For this review, take the finished solid that the model builds, in its own axes (mm). Give positions to 0.01 mm unless a question says otherwise; leave off trailing zeros. Loops run counter-clockwise (first coordinate to the right, second up) from the corner with the lowest first, then second, coordinate; pieces in that order, holes last. Notation, with made-up numbers: M 79,86 L 87,86 A26 ccw 87,103 Z; hole C 87,85 d9. An arc over 180 degrees is marked long. Use CSV: the item, a comma, the result in double quotes. Start each with the question number.
1. Insertion check: P1, Ø8, axis at x = 16.5, y = -30.5, coming from the -Z side; P2, Ø6, axis at x = 1.5, z = 7.5, coming from the -Y side; P3, Ø5, axis at y = 28.5, z = 10, coming from the -X side; P4, Ø8, axis at x = -27.5, y = -7.5, coming from the +Z side. Each pin has a flat end and moves straight along its axis. Give the tip position at first contact, or say it passes through.
2. Take a section at D-D, the plane y = -21. Write out the cut boundary in (x, z), and give its area (3 significant figures).
3. Take a section at A-A, the plane x = 0. Write out the cut boundary in (y, z) (3 decimals), and give its area (3 significant figures).
4. To check wall thickness, follow line 1 (Y direction, x = 0, z = 3.8) (3 decimals); line 2 (Z direction, x = 9.5, y = -13); line 3 (X direction, y = -36.5, z = 1.25). State the ranges of each line that lie inside material, in increasing order. Write a range as [from, to].
5. Take a section at C-C, the plane y = 2.5. Write out the cut boundary in (x, z).
from build123d import *

# Parameters (mm, degrees)
F1_DEPTH = 5.08
F2_R     = 3.6481835691
F3_DEPTH = 2.54
F4_R     = 1.6674700951
F5_DEPTH = 5.08
F6_R     = 8.255
F7_DEPTH = 25.4


with BuildPart() as f1:
    # F0 (on Top) → F1 (new body)
    with BuildSketch(Plane.XY):
        with BuildLine():
            ThreePointArc((37.7468732805, -5.1752833301), (38.0116158035, -2.5936584214), (38.1, 0))
            ThreePointArc((38.1, 0), (38.0577032994, 1.7947756344), (37.9309071088, 3.5855663298))
            Line((37.9309071088, 3.5855663298), (34.7138681986, 5.6416139149))
            Line((34.7138681986, 5.6416139149), (34.1414945044, -7.0454814325))
            Line((34.1414945044, -7.0454814325), (37.7468732805, -5.1752833301))
        make_face()
        with BuildLine():
            ThreePointArc((37.9309071088, 3.5855663298), (38.0577032994, 1.7947756344), (38.1, 0))
            ThreePointArc((38.1, 0), (38.0116158035, -2.5936584214), (37.7468732805, -5.1752833301))
            Line((37.7468732805, -5.1752833301), (45.4150282226, -1.1976239184))
            Line((45.4150282226, -1.1976239184), (37.9309071088, 3.5855663298))
        make_face()
        with BuildLine():
            Line((34.7138681986, 5.6416139149), (37.9309071088, 3.5855663298))
            ThreePointArc((37.9309071088, 3.5855663298), (36.4745263648, 11.0099467057), (33.5798171863, 18.0001632696))
            Line((33.5798171863, 18.0001632696), (31.7622793488, 14.3679527485))
            Line((31.7622793488, 14.3679527485), (24.7680518549, 24.9684613101))
            Line((24.7680518549, 24.9684613101), (28.5792054533, 25.1960118999))
            ThreePointArc((28.5792054533, 25.1960118999), (23.0370273887, 30.3464226737), (16.586412263, 34.3001593035))
            Line((16.586412263, 34.3001593035), (17.250953042, 30.2933173283))
            Line((17.250953042, 30.2933173283), (5.3616815377, 34.7582051315))
            Line((5.3616815377, 34.7582051315), (8.3112186861, 37.1824373052))
            ThreePointArc((8.3112186861, 37.1824373052), (0.8001669499, 38.0915966173), (-6.7424383934, 37.4986603029))
            Line((-6.7424383934, 37.4986603029), (-3.8496509884, 34.6476643207))
            Line((-3.8496509884, 34.6476643207), (-16.0926688901, 31.2714959807))
            Line((-16.0926688901, 31.2714959807), (-15.1313711312, 34.9664354444))
            ThreePointArc((-15.1313711312, 34.9664354444), (-21.7423300671, 31.2870753388), (-27.4959067505, 26.3739475992))
            Line((-27.4959067505, 26.3739475992), (-23.4798191861, 25.7677811734))
            Line((-23.4798191861, 25.7677811734), (-31.4001667715, 15.8401382443))
            Line((-31.4001667715, 15.8401382443), (-32.7942914728, 19.3944437094))
            ThreePointArc((-32.7942914728, 19.3944437094), (-35.9799959931, 12.5319546895), (-37.7468732805, 5.1752833301))
            Line((-37.7468732805, 5.1752833301), (-34.1414945044, 7.0454814325))
            Line((-34.1414945044, 7.0454814325), (-34.7138681986, -5.6416139149))
            Line((-34.7138681986, -5.6416139149), (-37.9309071088, -3.5855663298))
            ThreePointArc((-37.9309071088, -3.5855663298), (-36.4745263648, -11.0099467057), (-33.5798171863, -18.0001632696))
            Line((-33.5798171863, -18.0001632696), (-31.7622793488, -14.3679527485))
            Line((-31.7622793488, -14.3679527485), (-24.7680518549, -24.9684613101))
            Line((-24.7680518549, -24.9684613101), (-28.5792054533, -25.1960118999))
            ThreePointArc((-28.5792054533, -25.1960118999), (-23.0370273887, -30.3464226737), (-16.586412263, -34.3001593035))
            Line((-16.586412263, -34.3001593035), (-17.250953042, -30.2933173283))
            Line((-17.250953042, -30.2933173283), (-5.3616815377, -34.7582051315))
            Line((-5.3616815377, -34.7582051315), (-8.3112186861, -37.1824373052))
            ThreePointArc((-8.3112186861, -37.1824373052), (-0.8001669499, -38.0915966173), (6.7424383934, -37.4986603029))
            Line((6.7424383934, -37.4986603029), (3.8496509884, -34.6476643207))
            Line((3.8496509884, -34.6476643207), (16.0926688901, -31.2714959807))
            Line((16.0926688901, -31.2714959807), (15.1313711312, -34.9664354444))
            ThreePointArc((15.1313711312, -34.9664354444), (21.7423300671, -31.2870753388), (27.4959067505, -26.3739475992))
            Line((27.4959067505, -26.3739475992), (23.4798191861, -25.7677811734))
            Line((23.4798191861, -25.7677811734), (31.4001667715, -15.8401382443))
            Line((31.4001667715, -15.8401382443), (32.7942914728, -19.3944437094))
            ThreePointArc((32.7942914728, -19.3944437094), (35.9799959931, -12.5319546895), (37.7468732805, -5.1752833301))
            Line((37.7468732805, -5.1752833301), (34.1414945044, -7.0454814325))
            Line((34.1414945044, -7.0454814325), (34.7138681986, 5.6416139149))
        make_face()
        with BuildLine():
            Line((31.7622793488, 14.3679527485), (33.5798171863, 18.0001632696))
            ThreePointArc((33.5798171863, 18.0001632696), (31.2870753388, 21.7423300671), (28.5792054533, 25.1960118999))
            Line((28.5792054533, 25.1960118999), (24.7680518549, 24.9684613101))
            Line((24.7680518549, 24.9684613101), (31.7622793488, 14.3679527485))
        make_face()
        with BuildLine():
            ThreePointArc((28.5792054533, 25.1960118999), (31.2870753388, 21.7423300671), (33.5798171863, 18.0001632696))
            Line((33.5798171863, 18.0001632696), (37.4454753092, 25.7253857188))
            Line((37.4454753092, 25.7253857188), (28.5792054533, 25.1960118999))
        make_face()
        with BuildLine():
            Line((36.0375839551, -27.6631819246), (32.7942914728, -19.3944437094))
            ThreePointArc((32.7942914728, -19.3944437094), (30.3464226737, -23.0370273887), (27.4959067505, -26.3739475992))
            Line((27.4959067505, -26.3739475992), (36.0375839551, -27.6631819246))
        make_face()
        with BuildLine():
            ThreePointArc((27.4959067505, -26.3739475992), (30.3464226737, -23.0370273887), (32.7942914728, -19.3944437094))
            Line((32.7942914728, -19.3944437094), (31.4001667715, -15.8401382443))
            Line((31.4001667715, -15.8401382443), (23.4798191861, -25.7677811734))
            Line((23.4798191861, -25.7677811734), (27.4959067505, -26.3739475992))
        make_face()
        with BuildLine():
            Line((17.250953042, 30.2933173283), (16.586412263, 34.3001593035))
            ThreePointArc((16.586412263, 34.3001593035), (12.5319546895, 35.9799959931), (8.3112186861, 37.1824373052))
            Line((8.3112186861, 37.1824373052), (5.3616815377, 34.7582051315))
            Line((5.3616815377, 34.7582051315), (17.250953042, 30.2933173283))
        make_face()
        with BuildLine():
            ThreePointArc((8.3112186861, 37.1824373052), (12.5319546895, 35.9799959931), (16.586412263, 34.3001593035))
            Line((16.586412263, 34.3001593035), (15.1730235525, 42.8221723852))
            Line((15.1730235525, 42.8221723852), (8.3112186861, 37.1824373052))
        make_face()
        with BuildLine():
            Line((12.8950074891, -43.5623446725), (15.1313711312, -34.9664354444))
            ThreePointArc((15.1313711312, -34.9664354444), (11.0099467057, -36.4745263648), (6.7424383934, -37.4986603029))
            Line((6.7424383934, -37.4986603029), (12.8950074891, -43.5623446725))
        make_face()
        with BuildLine():
            ThreePointArc((6.7424383934, -37.4986603029), (11.0099467057, -36.4745263648), (15.1313711312, -34.9664354444))
            Line((15.1313711312, -34.9664354444), (16.0926688901, -31.2714959807))
            Line((16.0926688901, -31.2714959807), (3.8496509884, -34.6476643207))
            Line((3.8496509884, -34.6476643207), (6.7424383934, -37.4986603029))
        make_face()
        with BuildLine():
            Line((-3.8496509884, 34.6476643207), (-6.7424383934, 37.4986603029))
            ThreePointArc((-6.7424383934, 37.4986603029), (-11.0099467057, 36.4745263648), (-15.1313711312, 34.9664354444))
            Line((-15.1313711312, 34.9664354444), (-16.0926688901, 31.2714959807))
            Line((-16.0926688901, 31.2714959807), (-3.8496509884, 34.6476643207))
        make_face()
        with BuildLine():
            ThreePointArc((-15.1313711312, 34.9664354444), (-11.0099467057, 36.4745263648), (-6.7424383934, 37.4986603029))
            Line((-6.7424383934, 37.4986603029), (-12.8950074891, 43.5623446725))
            Line((-12.8950074891, 43.5623446725), (-15.1313711312, 34.9664354444))
        make_face()
        with BuildLine():
            Line((-15.1730235525, -42.8221723852), (-8.3112186861, -37.1824373052))
            ThreePointArc((-8.3112186861, -37.1824373052), (-12.5319546895, -35.9799959931), (-16.586412263, -34.3001593035))
            Line((-16.586412263, -34.3001593035), (-15.1730235525, -42.8221723852))
        make_face()
        with BuildLine():
            ThreePointArc((-16.586412263, -34.3001593035), (-12.5319546895, -35.9799959931), (-8.3112186861, -37.1824373052))
            Line((-8.3112186861, -37.1824373052), (-5.3616815377, -34.7582051315))
            Line((-5.3616815377, -34.7582051315), (-17.250953042, -30.2933173283))
            Line((-17.250953042, -30.2933173283), (-16.586412263, -34.3001593035))
        make_face()
        with BuildLine():
            Line((-23.4798191861, 25.7677811734), (-27.4959067505, 26.3739475992))
            ThreePointArc((-27.4959067505, 26.3739475992), (-30.3464226737, 23.0370273887), (-32.7942914728, 19.3944437094))
            Line((-32.7942914728, 19.3944437094), (-31.4001667715, 15.8401382443))
            Line((-31.4001667715, 15.8401382443), (-23.4798191861, 25.7677811734))
        make_face()
        with BuildLine():
            ThreePointArc((-32.7942914728, 19.3944437094), (-30.3464226737, 23.0370273887), (-27.4959067505, 26.3739475992))
            Line((-27.4959067505, 26.3739475992), (-36.0375839551, 27.6631819246))
            Line((-36.0375839551, 27.6631819246), (-32.7942914728, 19.3944437094))
        make_face()
        with BuildLine():
            Line((-37.4454753092, -25.7253857188), (-28.5792054533, -25.1960118999))
            ThreePointArc((-28.5792054533, -25.1960118999), (-31.2870753388, -21.7423300671), (-33.5798171863, -18.0001632696))
            Line((-33.5798171863, -18.0001632696), (-37.4454753092, -25.7253857188))
        make_face()
        with BuildLine():
            ThreePointArc((-33.5798171863, -18.0001632696), (-31.2870753388, -21.7423300671), (-28.5792054533, -25.1960118999))
            Line((-28.5792054533, -25.1960118999), (-24.7680518549, -24.9684613101))
            Line((-24.7680518549, -24.9684613101), (-31.7622793488, -14.3679527485))
            Line((-31.7622793488, -14.3679527485), (-33.5798171863, -18.0001632696))
        make_face()
        with BuildLine():
            Line((-34.1414945044, 7.0454814325), (-37.7468732805, 5.1752833301))
            ThreePointArc((-37.7468732805, 5.1752833301), (-38.0915966173, 0.8001669499), (-37.9309071088, -3.5855663298))
            Line((-37.9309071088, -3.5855663298), (-34.7138681986, -5.6416139149))
            Line((-34.7138681986, -5.6416139149), (-34.1414945044, 7.0454814325))
        make_face()
        with BuildLine():
            ThreePointArc((-37.9309071088, -3.5855663298), (-38.0915966173, 0.8001669499), (-37.7468732805, 5.1752833301))
            Line((-37.7468732805, 5.1752833301), (-45.4150282226, 1.1976239184))
            Line((-45.4150282226, 1.1976239184), (-37.9309071088, -3.5855663298))
        make_face()
    extrude(amount=F1_DEPTH)

    # F2 (on face) → F3 (join)
    with BuildSketch(Plane.XY.offset(5.08)):
        with Locations((-23.9648092538, 18.6180789024)):
            Circle(F2_R)
    extrude(amount=F3_DEPTH)

    # F4 (on face) → F5 (join)
    with BuildSketch(Plane.XY.offset(7.62)):
        with Locations((-23.9648092538, 18.6180789024)):
            Circle(F4_R)
    extrude(amount=F5_DEPTH)

    # F6 (on face) → F7 (cut)
    with BuildSketch(Plane.XY.offset(5.08)):
        Circle(F6_R)
    extrude(amount=-F7_DEPTH, mode=Mode.SUBTRACT)


solid = f1.part
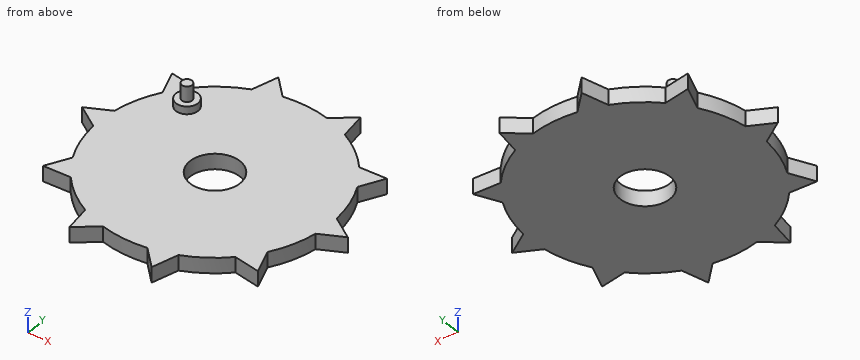
Result set:
1,P1,"z = 0"
1,P2,"y = -38.1"
1,P3,"through"
1,P4,"z = 5.08"
2,outline,"M -35.08,0 L 33.42,0 L 33.42,5.08 L -35.08,5.08 Z"
2,area,"348 mm2"
3,outline,"M -38.1,0 L -8.255,0 L -8.255,5.08 L -38.1,5.08 Z; M 8.255,0 L 38.1,0 L 38.1,5.08 L 8.255,5.08 Z"
3,area,"303 mm2"
4,line 1,"[-38.1, -8.255], [8.255, 38.1]"
4,line 2,"[0, 5.08]"
4,line 3,"[-16.22, 14.73]"
5,outline,"M -42.9,0 L -7.87,0 L -7.87,5.08 L -42.9,5.08 Z; M 7.87,0 L 39.63,0 L 39.63,5.08 L 7.87,5.08 Z"
